Autodesk Inventor part; units mm, degrees
ref_plane "YZ Plane" through (0, 0, 0) normal (1, 0, 0) x (0, 1, 0)
ref_plane "XZ Plane" through (0, 0, 0) normal (0, 1, 0) x (-1, 0, 0)
ref_plane "XY Plane" through (0, 0, 0) normal (0, 0, 1) x (1, 0, 0)
sketch "Sketch1" plane through (0, 0, 0) normal (0, 0, 1) x (1, 0, 0)
  circle A0 centre (12.5, 11.5) radius 1.6
  line L0 (0, 0) -> (18, 0)
  line L1 (0, 0) -> (0, 3)
  arc A1 (18, 11.5) -> (7.7369, 14.25) centre (12.5, 11.5) ccw
  line L2 (12.5, 11.5) -> (7.7369, 14.25) construction
  line L3 (12.5, 11.5) -> (18, 11.5) construction
  line L4 (7.7369, 14.25) -> (0, 3)
  line L5 (18, 11.5) -> (18, 0)
  dimension "d17" = 3
  dimension "d19" = 11.5
  dimension "d23" = 90
  dimension "d25" = 12.5
  dimension "d31" = 5.5
  dimension "d32" = 150
extrude "Extrusion1" add sketch "Sketch1" along normal blind 4.5
sketch "Sketch4" plane through (0, 0, 4.5) normal (0, 0, 1) x (1, 0, 0)
  line L0 (0, 3) -> (0, 0)
  line L1 (18, 0) -> (18, 3)
  line L2 (0, 0) -> (18, 0)
  line L3 (18, 0) -> (18, 3)
  line L4 (18, 3) -> (0, 3)
  line L5 (0, 3) -> (0, 0)
  line L6 (18, 0) -> (18, 11.5)
extrude "Extrusion2" add sketch "Sketch4" along normal blind 4.5
sketch "Sketch5" plane through (0, 0, 0) normal (0, -1, 0) x (1, 0, 0)
  circle A0 centre (5, 4.8) radius 0.5
  circle A1 centre (15, 4.8) radius 0.5
  line L0 (0, 0) -> (18, 0)
  point P0 (20.0001, 0)
  dimension "d13" = 1
  dimension "d14" = 1
  dimension "d38" = 4.8
  dimension "d39" = 4.8
extrude "Extrusion3" cut sketch "Sketch5" against normal through all
sketch "Sketch6" plane through (0, 3, 9) normal (0, 1, 0) x (1, 0, 0)
  circle A0 centre (5, 4.2) radius 0.5
  circle A1 centre (5, 4.2) radius 3
  circle A2 centre (15, 4.2) radius 0.5
  circle A3 centre (15, 4.2) radius 3
  line L0 (0, 9) -> (18, 9)
  point P0 (20.0001, 9)
  dimension "d34" = 6
  dimension "d35" = 6
  dimension "d40" = 4.8
  dimension "d41" = 4.8
extrude "Extrusion4" cut sketch "Sketch6" along normal up to next
sketch "Sketch7" plane through (0, 0, 0) normal (0, -1, 0) x (1, 0, 0)
  line L0 (0, 0) -> (0, 9)
  line L1 (2.042, 0) -> (0, 0)
  line L2 (0, 0) -> (0, 9)
  line L3 (0, 9) -> (2.042, 9)
  line L4 (2.042, 9) -> (2.042, 0)
extrude "Extrusion5" cut sketch "Sketch7" against normal up to next
properties part number "lower_deck_shaft_mount_v2_printing_inna_plaszczyzna_jako_baza"
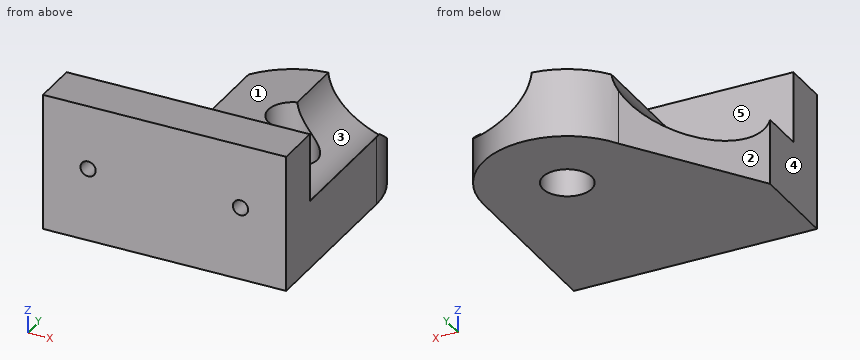
Input: part model. Units: mm. Frame: model coordinates. Face numbers are marked on the shaded views. A direction names the side the tool comes from. Round coordinates to 2 decimals unless told otherwise and drop trailing zeros. Write each loop counter-clockwise with the first axis right and the second up, starting at its lowest first coordinate (ties: lowest second). Pieces come first, ordered by that corner, then holes.
1) Draft query along X for the marked faces 1, 2 and 3. Return one class per face: pulls with the +X half, pulls with the -X half, needs draft (parallel to the pull), parting line crosses it, or undercut.
2) Contact query for flat-ended pins moving along their axis: P1, Ø2.5, axis at x = 12.5, y = 11.5, coming from the -Z side; P2, Ø5, axis at x = 10, z = 3.5, coming from the +Y side; P3, Ø4.5, axis at x = 9, y = 12.5, coming from the +Z side; P4, Ø2, axis at x = 6, z = 6, coming from the +Y side. Output: stop coordinate, or through.
3) Ray query, L1, parallel to Z at x = 5, y = 1.75; L2, parallel to Y at x = 12.5, z = 2.9; L3, parallel to Y at x = 15.75, z = 3.75. Return the intervals inside material, ascending.
4) Cut plane A-A (z = 4.8). Return the cut outline in (x, y), then the cut area to 3 significant figures.
5) Cut plane B-B (x = 5). Return the cut outline in (y, z).
6) Reachability of the marked faces 4 and 5 from +Z, -Z, +X, -X, +Y, -Y: full face, straight path, thin tool, end or side. Return the list, or none.
7) Cut plane D-D (z = 1.5). Return the cut outline in (x, y), then the cut area to 3 significant figures.
Geometry says:
1. face 1: needs draft
1. face 2: pulls with the -X half
1. face 3: undercut
2. P1: passes through
2. P2: stops at y = 17
2. P3: stops at z = 4.5
2. P4: stops at y = 3
3. L1: z = 0 to 4.3, 5.3 to 9
3. L2: y = 0 to 9.9, 13.1 to 17
3. L3: y = 0 to 3
4. outline: (2.04, 0) - (4.5, 0) - (4.5, 3) - (2.04, 3) - close; (5.5, 0) - (14.5, 0) - (14.5, 3) - (5.5, 3) - close; (15.5, 0) - (18, 0) - (18, 3) - (15.5, 3) - close
4. area: 41.9 mm2
5. outline: (0, 0) - (10.27, 0) - (10.27, 1.8) - (3, 1.8) - (3, 4.3) - (0, 4.3) - close; (0, 5.3) - (3, 5.3) - (3, 9) - (0, 9) - close
6. face 4: +Z, -Z, -X, +Y, -Y
6. face 5: +Z, +Y
7. outline: (2.04, 0) - (18, 0) - (18, 11.5) arc R5.5 ccw to (7.74, 14.25) - (2.04, 5.97) - close; hole circle Ø3.2 at (12.5, 11.5)
7. area: 214 mm2
